Design review of the part shown in the three views and the two pictorial views. Dimensions are in mm from the part's minimum x, y and z. Give positions to 0.01 mm unless a question says otherwise; leave off trailing zeros. Order: outer loops, then holes, each group sorted by start corner. A loop starts at its lowest first (then second) coordinate and runs counter-clockwise, first axis right, second up.
Item 1: For probe 1 along Y at (x, z) = (30, 2.15); probe 2 along X at (y, z) = (3.5, 3.5); probe 3 along X at (y, z) = (4.25, 3.95), list the stretches that pass through material, from the lowest coordinate up.
Item 2: Consider section C-C (y = 2.25). Give the boundary of the cut face in (x, z).
Item 3: For P1, Ø1, axis at y = 5, z = 2, coming from the -X side; P2, Ø2, axis at y = 2.5, z = 4, coming from the +X side, all flat-tipped, find the tip position at first contact; note any pin that passes through.
Item 4: Consider section A-A (z = 4.1). Give the boundary of the cut face in (x, y).
Item 5: Consider section B-B (x = 30). Give the boundary of the cut face in (y, z).
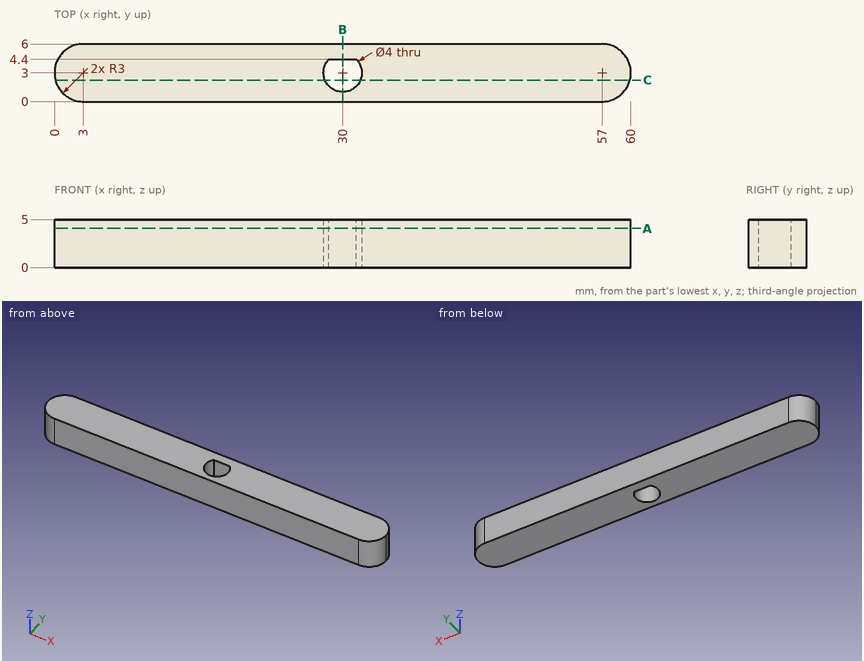
Resolved:
1. probe 1: y = 0 to 1, 4.4 to 6
1. probe 2: x = 0.04 to 28.06, 31.94 to 59.96
1. probe 3: x = 0.27 to 28.44, 31.56 to 59.73
2. outline: (0.1, 0) - (28.15, 0) - (28.15, 5) - (0.1, 5) - close; (31.85, 0) - (59.9, 0) - (59.9, 5) - (31.85, 5) - close
3. P1: stops at x = 0.4
3. P2: stops at x = 60
4. outline: (0, 3) arc R3 ccw to (3, 0) - (57, 0) arc R3 ccw to (60, 3) arc R3 ccw to (57, 6) - (3, 6) arc R3 ccw to start; hole (28.57, 4.4) arc R2 ccw (long way) to (31.43, 4.4) - close
5. outline: (0, 0) - (1, 0) - (1, 5) - (0, 5) - close; (4.4, 0) - (6, 0) - (6, 5) - (4.4, 5) - close
